Build history of the part. All positions in model axes, mm. A direction names the side the tool comes from. Round coordinates to 2 decimals unless told otherwise and drop trailing zeros. Loops run counter-clockwise (first coordinate to the right, second up) from the corner with the lowest first, then second, coordinate; pieces in that order, holes last. Notation, with made-up numbers: (33, 62) - (39, 62) arc R24 cw to (39, 74) - close; hole circle Ø1 at (-36.5, 9). An arc over 180 degrees is marked (long way). Answer as CSV lines item,"result". Start each with the question number.
```python
from build123d import *

# Parameters (mm, degrees)
BOSS_EXTRUDE1_DEPTH = 6.35


with BuildPart() as part:
    # Sketch1 → Boss-Extrude1 (new body)
    with BuildSketch(Plane.XY):
        Polygon((25.4, 0), (12.7, 299.72), (8.89, 299.72), (8.89, 306.07), (5.08, 306.07), (5.08, 299.72), (1.7, 299.72), (1.7, 296.926), (2.97, 296.926), (2.97, 294.894), (1.7, 294.894), (1.7, 293.37), (-1.7, 293.37), (-1.7, 294.894), (-2.97, 294.894), (-2.97, 296.926), (-1.7, 296.926), (-1.7, 299.72), (-5.08, 299.72), (-5.08, 306.07), (-8.89, 306.07), (-8.89, 299.72), (-12.7, 299.72), (-25.4, 0), (-20.32, 0), (-20.32, -6.35), (-17.526, -6.35), (-17.526, 0), (17.526, 0), (17.526, -6.35), (20.32, -6.35), (20.32, 0), align=None)
        with BuildLine():
            Line((-8.89, 150.297214184), (8.89, 150.297214184))
            Line((8.89, 150.297214184), (8.89, 169.347214184))
            ThreePointArc((8.89, 169.347214184), (0, 178.237214184), (-8.89, 169.347214184))
            Line((-8.89, 169.347214184), (-8.89, 150.297214184))
        make_face(mode=Mode.SUBTRACT)
    extrude(amount=BOSS_EXTRUDE1_DEPTH)


solid = part.part
```
Q1. Tool access for faces 4 (the flat face through (5.08, 303, 3)), 5 (the flat face through (8.89, 160, 3)), 6 (the flat face through (8.89, 303, 3)), 7 (the flat face through (-17.526, -3, 3)): list every direction of +Z, -Z, +X, -X, +Y, -Y with a clear straight run to the whole face (end or side of a thin tool).
Q2. Wall check: probe 1 along Y at (x, z) = (2.5, 3.25); probe 2 along Y at (x, z) = (10, 5.5); probe 3 along X at (y, z) = (162.5, 3.75). Give the ranges that are in metal, low to high. Write a range as [from, to].
Q3. Pin check, flat tips, straight feed: pin 1 Ø0.6 at (x, z) = (2.5, 1.5) entering from -Y; pin 2 Ø2 at (y, z) = (297.5, 3.5) entering from +X; pin 3 Ø3 at (y, z) = (45.5, 3) entering from -X. Stop position of each tip, or through.
Q4. Band-saw the part on A-A, the plane y = 63.5. List the corners of the cut face in (x, z), then the cut area to 3 significant figures.
Q5. Two-plate mould, pull along Y, no slides. Class faces 1 (the flat face through (0, 117, 6.35)), 2 (the flat face through (-18.96, 151.96, 3.13)), 3 (the flat face through (0, 150.297, 3)): released by +Y, released by -Y, zero draft, split by the parting line, or undercut.
Reported:
1,face 4,"+Z, -Z, +Y"
1,face 5,"+Z, -Z"
1,face 6,"+Z, -Z, +X, +Y"
1,face 7,"+Z, -Z, -Y"
2,probe 1,"y = [0, 150.3], [177.88, 294.89], [296.93, 299.72]"
2,probe 2,"y = [0, 299.72]"
2,probe 3,"x = [-18.51, -8.89], [8.89, 18.51]"
3,pin 1,"stops at y = 0"
3,pin 2,"stops at x = 12.84"
3,pin 3,"stops at x = -23.54"
4,outline,"(-22.71, 0) - (22.71, 0) - (22.71, 6.35) - (-22.71, 6.35) - close"
4,area,"288 mm2"
5,face 1,"zero draft"
5,face 2,"released by +Y"
5,face 3,"undercut"
